Work out the finished part from the listing and answer in its coordinate system (mm). Face numbers are marked on the shaded views. A direction names the side the tool comes from. Coordinates: 2 decimals unless noted, no trailing zeros. Write each loop counter-clockwise with the first axis right and the second up, starting at its lowest first coordinate (ties: lowest second). Pieces come first, ordered by that corner, then holes. Notation, with made-up numbers: M -33,29.5 L 15,29.5 A17 cw 15,52.5 Z; hole C -22.75,62 d10. An arc over 180 degrees is marked long. Use CSV: the item, a comma, the result in double quotes.
Autodesk Inventor part; units mm, degrees
ref_plane "YZ Plane" through (0, 0, 0) normal (1, 0, 0) x (0, 1, 0)
ref_plane "XZ Plane" through (0, 0, 0) normal (0, 1, 0) x (-1, 0, 0)
ref_plane "XY Plane" through (0, 0, 0) normal (0, 0, 1) x (1, 0, 0)
sketch "Esboço1" plane through (0, 0, 0) normal (0, 1, 0) x (-1, 0, 0)
  line L0 (6, 5) -> (-6, 5)
  line L1 (-6, 5) -> (-6, -5)
  line L2 (-6, -5) -> (6, -5)
  line L3 (6, -5) -> (6, 5)
  line L4 (6, 5) -> (-6, -5) construction
  line L5 (-6, 5) -> (6, -5) construction
  point P0 (0, 0)
  dimension "d0" = 12
  dimension "d1" = 10
extrude "Extrusão1" add sketch "Esboço1" along normal blind 0.8
fillet "Arredondamento1" radius 1 4 edges at (-6, 0.4, 5) (6, 0.4, 5) (6, 0.4, -5) (-6, 0.4, -5)
sketch "Esboço2" plane through (0, 0.8, 0) normal (0, 1, 0) x (1, 0, 0)
  circle A0 centre (0, 0) radius 2
  circle A1 centre (0, 0) radius 1.5
  dimension "d5" = 4
  dimension "d6" = 3
extrude "Extrusão2" add sketch "Esboço2" along normal blind 0.7
extrude "Extrusão3" cut sketch "Esboço2" against normal blind 0.8 contours A1
sketch "Esboço3" plane through (0, 0.8, 0) normal (0, 1, 0) x (1, 0, 0)
  circle A0 centre (4.5, 0) radius 0.8
  circle A1 centre (0, 0) radius 1.5
  line L0 (0, -1.5) -> (0, 1.5)
  circle A2 centre (-4.5, 0) radius 0.8
  circle A3 centre (0, 0) radius 1.5
  dimension "d11" = 1.6
extrude "Extrusão4" cut sketch "Esboço3" against normal blind 0.8 contours A0 | A2
sketch "Esboço4" plane through (0, 0.8, 0) normal (0, 1, 0) x (1, 0, 0)
  circle A0 centre (-3.0146, 1.9633) radius 0.45
  circle A1 centre (0, 0) radius 2
  line L0 (5, 5) -> (-5, 5)
  line L1 (-5, -5) -> (5, -5)
  circle A2 centre (3.0146, -1.9633) radius 0.45
  dimension "d14" = 0.9
  dimension "d15" = 0.9
extrude "Extrusão5" cut sketch "Esboço4" against normal blind 0.8 contours A0 | A2
sketch "Esboço5" plane through (0, 0.8, 0) normal (0, 1, 0) x (1, 0, 0)
  circle A0 centre (3.8014, 2.7994) radius 1.25
  circle A1 centre (-3.8014, -2.7994) radius 1.25
  circle A2 centre (3.8014, 2.7994) radius 0.75
  circle A3 centre (-3.8014, -2.7994) radius 0.75
  point P0 (0, 0)
  dimension "d18" = 2.5
  dimension "d19" = 2.5
  dimension "d22" = 1.5
  dimension "d30" = 1.5
extrude "Extrusão6" cut sketch "Esboço5" against normal blind 0.4 contours A0 | A1 | A2 | A3
extrude "Extrusão7" cut sketch "Esboço5" against normal blind 10 contours A2 | A3
sketch "Esboço6" plane through (0, 0, 0) normal (0, -1, 0) x (1, 0, 0)
  circle A0 centre (-3.8014, 2.7994) radius 0.75
  circle A1 centre (-3.8014, 2.7994) radius 1.5
  circle A2 centre (3.8014, -2.7994) radius 0.75
  circle A3 centre (3.8014, -2.7994) radius 1.5
  point P0 (0, 0)
  dimension "d26" = 3
  dimension "d27" = 3
extrude "Extrusão8" add sketch "Esboço6" along normal blind 4.6
thread "Rosca1"
thread "Rosca2"
sketch "Esboço10" plane through (0, 0, 0) normal (0, -1, 0) x (1, 0, 0)
  circle A0 centre (0, 0) radius 2
  circle A1 centre (0, 0) radius 1.5
extrude "Extrusão9" add sketch "Esboço10" along normal blind 0.1
properties part number "Chapa Superior"
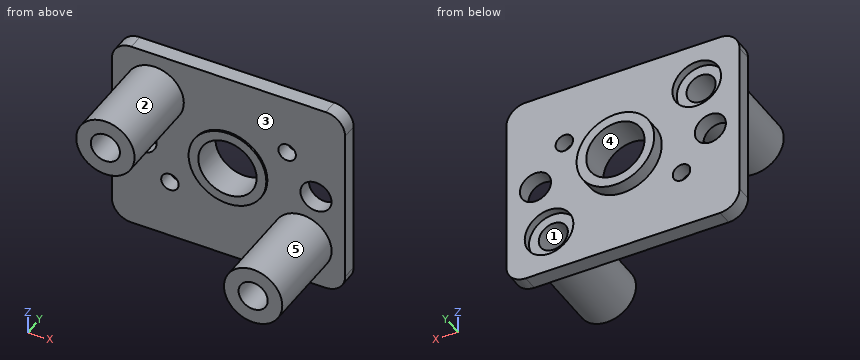
Item 1: A tool of negligible diameter and unlimited length cuts with its end or side. For the marked faces 4 and 5, from which of +Z, -Z, +X, -X, +Y, -Y can it reach the whole face along a straight path? Write none if from no direction.
Answer:
face 4,"+Y, -Y"
face 5,"-Y"
Item 2: Consider probe 1 along X at (y, z) = (0.2, 0); probe 2 along Z at (x, y) = (-3.75, -3.5); probe 3 along X at (y, z) = (-2.75, 2.75). Determine where each line is inside the solid, lowest interval first.
Answer:
probe 1,"x = -6 to -5.3, -3.7 to -1.5, 1.5 to 3.7, 5.3 to 6"
probe 2,"z = 1.3 to 2.05, 3.55 to 4.3"
probe 3,"x = -5.3 to -4.55, -3.05 to -2.3"
Item 3: Given pin 1 (2 mm diameter, centred on x = 3.8, z = -2.8, fed in from +Y); pin 2 (1.8 mm diameter, centred on x = 4.5, z = 0, fed in from -Y); pin 3 (2 mm diameter, centred on x = -0.5, z = 0.5, fed in from -Y), each flat-ended and moving along its own axis, determine where each tip first touches the part or whether it passes through.
Answer:
pin 1,"stops at y = 0.4"
pin 2,"stops at y = 0"
pin 3,"stops at y = -0.1"
Item 4: The part is cut by section B-B (z = 0). Write down the section's boundary in (x, y).
Answer:
outline,"M -6,0 L -5.3,0 L -5.3,0.8 L -6,0.8 Z; M -3.7,0 L -2,0 L -2,-0.1 L -1.5,-0.1 L -1.5,1.5 L -2,1.5 L -2,0.8 L -3.7,0.8 Z; M 1.5,-0.1 L 2,-0.1 L 2,0 L 3.7,0 L 3.7,0.8 L 2,0.8 L 2,1.5 L 1.5,1.5 Z; M 5.3,0 L 6,0 L 6,0.8 L 5.3,0.8 Z"
Item 5: The part is cut by section D-D (z = -2.25). Write down the section's boundary in (x, y).
Answer:
outline,"M -6,0 L -3.36,0 L -3.36,0.8 L -6,0.8 Z; M -2.67,0 L 2.41,0 L 2.41,-4.6 L 3.29,-4.6 L 3.29,0.4 L 2.68,0.4 L 2.68,0.8 L -2.67,0.8 Z; M 4.31,-4.6 L 5.2,-4.6 L 5.2,0 L 6,0 L 6,0.8 L 4.92,0.8 L 4.92,0.4 L 4.31,0.4 Z"
Item 6: The part is cut by section A-A (x = 0). Write down the section's boundary in (y, z), then the cut area to 3 significant figures.
Answer:
outline,"M -0.1,-2 L 0,-2 L 0,-5 L 0.8,-5 L 0.8,-2 L 1.5,-2 L 1.5,-1.5 L -0.1,-1.5 Z; M -0.1,1.5 L 1.5,1.5 L 1.5,2 L 0.8,2 L 0.8,5 L 0,5 L 0,2 L -0.1,2 Z"
area,"6.40 mm2"
Item 7: For a pull along Z with two mould halves and no side action, classify the marked faces 1, 2 and 3 as released by +Z, released by -Z, zero draft, split by the parting line, or undercut.
Answer:
face 1,"undercut"
face 2,"split by the parting line"
face 3,"zero draft"
Item 8: The part is cut by section C-C (z = -1). Write down the section's boundary in (x, y).
Answer:
outline,"M -6,0 L -1.73,0 L -1.73,-0.1 L -1.12,-0.1 L -1.12,1.5 L -1.73,1.5 L -1.73,0.8 L -6,0.8 Z; M 1.12,-0.1 L 1.73,-0.1 L 1.73,0 L 6,0 L 6,0.8 L 1.73,0.8 L 1.73,1.5 L 1.12,1.5 Z"
